Geometry check sheet. Reference: drawing and pictorial views, mm from the part's lowest x, y, z. Round coordinates to 2 decimals unless told otherwise and drop trailing zeros. Loops run counter-clockwise (first coordinate to the right, second up) from the corner with the lowest first, then second, coordinate; pieces in that order, holes last. Notation, with made-up numbers: (88, 63.25) -> (136, 63.25) arc R32 ccw to (136, 90.25) -> close; hole circle Ø2 at (80.5, 58.25). An arc over 180 degrees is marked (long way). Write item = value, one per line.
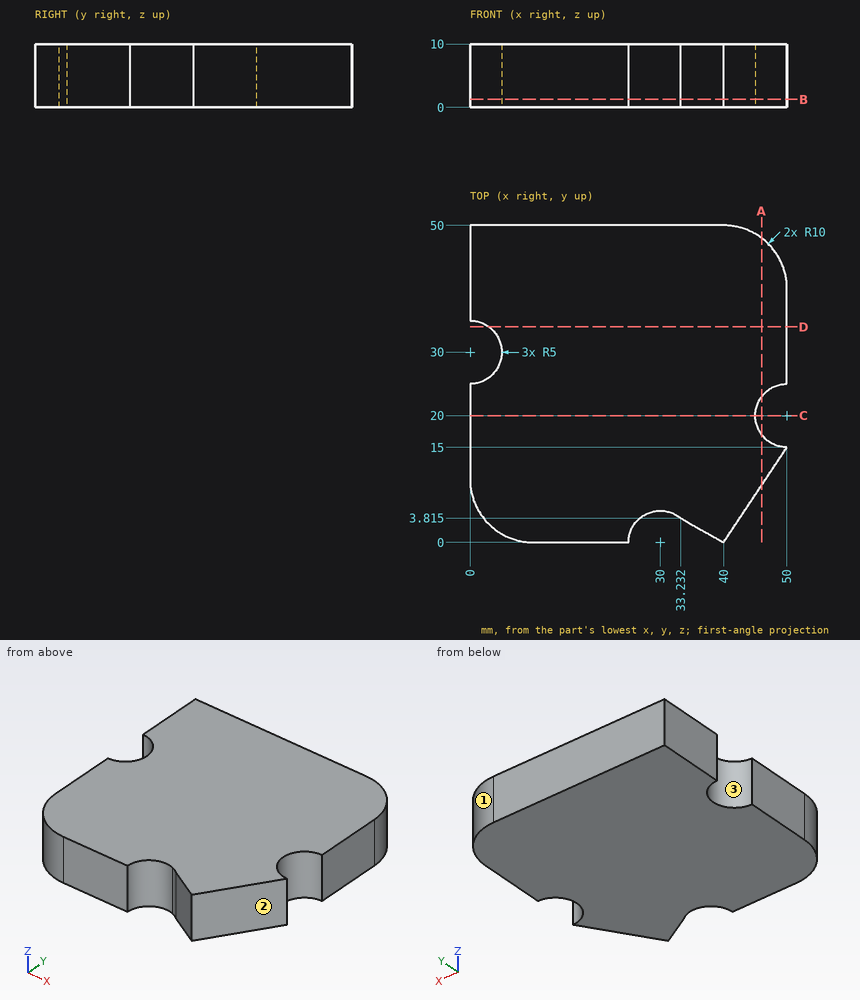
(1) Material ranges on probe 1 along Y at (x, z) = (46.5, 3.5); probe 2 along Y at (x, z) = (4.5, 2); probe 3 along Y at (x, z) = (9.5, 8), recorded low to high. Write a range as from..to.
Filled sheet:
probe_1 = 9.75..16.43, 23.57..47.6
probe_2 = 1.65..27.82, 32.18..50
probe_3 = 0.01..50
(2) Sectioned sample at C-C, the plane y = 20. Record the cut outline in (x, z), and give its area (3 significant figures).
Filled sheet:
outline = (0, 0) -> (45, 0) -> (45, 10) -> (0, 10) -> close
area = 450 mm2
(3) Sectioned sample at D-D, the plane y = 34. Record the cut outline in (x, z), and give its area (3 significant figures).
Filled sheet:
outline = (3, 0) -> (50, 0) -> (50, 10) -> (3, 10) -> close
area = 470 mm2
(4) Sectioned sample at B-B, the plane z = 1.25. Record the cut outline in (x, y) (1 decimal), and give its area (3 significant figures).
Filled sheet:
outline = (0, 10) arc R10 ccw to (10, 0) -> (25, 0) arc R5 cw to (31.6, 4.7) arc R5 cw to (33.2, 3.8) -> (40, 0) -> (50, 15) arc R5 cw to (50, 25) -> (50, 40) arc R10 ccw to (40, 50) -> (0, 50) -> (0, 35) arc R5 cw to (0, 25) -> close
area = 2,260 mm2
(5) Sectioned sample at A-A, the plane x = 46. Record the cut outline in (y, z).
Filled sheet:
outline = (9, 0) -> (17, 0) -> (17, 10) -> (9, 10) -> close; (23, 0) -> (48, 0) -> (48, 10) -> (23, 10) -> close
(6) Draft check along Y on the marked faces 1, 2 and 3. Enter one of: released by +Y, released by -Y, zero draft, split by the parting line, or undercut.
Filled sheet:
face_1 = released by +Y
face_2 = released by -Y
face_3 = undercut
(7) Go/stop test with a flat-tipped pin: pin 1 Ø6 at (x, y) = (6.5, 33) entering from -Z. Record where the tip stops, or that it passes through.
Filled sheet:
pin_1 = 0
